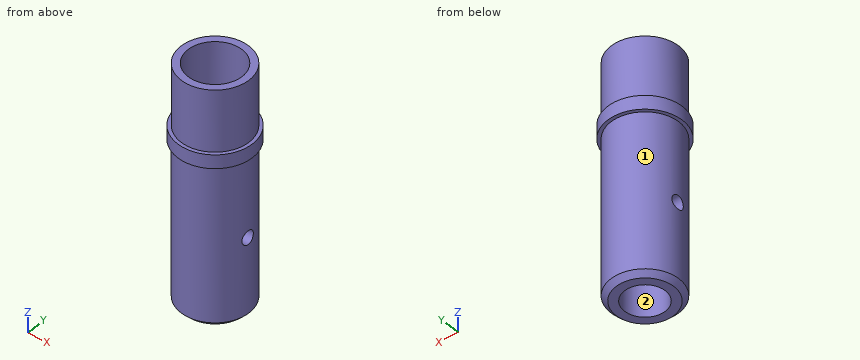
from build123d import *

# Parameters (mm, degrees)
SZKIC1_R                    = 10
SZKIC1_R_2                  = 7.9375
DODANIE_WYCI_GNI_CIE1_DEPTH = 18
SZKIC2_R                    = 11
SZKIC2_R_2                  = 7.9375
DODANIE_WYCI_GNI_CIE2_DEPTH = 4
SZKIC3_R                    = 10
SZKIC3_R_2                  = 6
DODANIE_WYCI_GNI_CIE3_DEPTH = 47
SFAZOWANIE1_SIZE            = 1.5
SZKIC6_R                    = 2
WYTNIJ_WYCI_GNI_CIE1_DEPTH  = 15


with BuildPart() as part:
    # Szkic1 → Dodanie-wyciągnięcie1 (new body)
    with BuildSketch(Plane.XY):
        Circle(SZKIC1_R)
        Circle(SZKIC1_R_2, mode=Mode.SUBTRACT)
    extrude(amount=DODANIE_WYCI_GNI_CIE1_DEPTH)

    # Szkic2 → Dodanie-wyciągnięcie2 (add)
    with BuildSketch(Plane(origin=(0, 0, 0), x_dir=(-1, 0, 0), z_dir=(0, 0, -1))):
        Circle(SZKIC2_R)
        Circle(SZKIC2_R_2, mode=Mode.SUBTRACT)
    extrude(amount=DODANIE_WYCI_GNI_CIE2_DEPTH)

    # Szkic3 → Dodanie-wyciągnięcie3 (add)
    with BuildSketch(Plane(origin=(0, 0, -4), x_dir=(-1, 0, 0), z_dir=(0, 0, -1))):
        Circle(SZKIC3_R)
        Circle(SZKIC3_R_2, mode=Mode.SUBTRACT)
    extrude(amount=DODANIE_WYCI_GNI_CIE3_DEPTH)

    # Sfazowanie1
    sfazowanie1_edges = [part.edges().sort_by_distance(p)[0] for p in [
        (10, 0, -51),
    ]]
    chamfer(sfazowanie1_edges, length=SFAZOWANIE1_SIZE)

    # Szkic6 → Wytnij-wyciągnięcie1 (cut, symmetric)
    with BuildSketch(Plane(origin=(0, 0, 0), x_dir=(0, 0, -1), z_dir=(1, 0, 0))):
        with Locations((27.5, 0)):
            Circle(SZKIC6_R)
    extrude(amount=WYTNIJ_WYCI_GNI_CIE1_DEPTH, both=True, mode=Mode.SUBTRACT)


solid = part.part
Verification items for the finished model (mm, model axes). Face numbers are marked on the shaded views. Coordinates: 2 decimals unless noted, no trailing zeros. Order: outer loops, then holes, each group sorted by start corner. A loop starts at its lowest first (then second) coordinate and runs counter-clockwise, first axis right, second up. Notation, with made-up numbers: (66.25, -38) -> (107.25, -38) arc R31 cw to (107.25, -12) -> close; hole circle Ø8 at (58.25, -39). An arc over 180 degrees is marked (long way). Put each result on its own line as item: value. Start each with the question number.
1. Cross-section at A-A, the plane y = 0. Count the separate pieces of the cut face and the enclosed holes in it, then the cut area to 4 significant figures.
2. Cross-section at C-C, the plane z = -27.5. Record the boundary of the cut face in (x, y), then the cut area to 3 significant figures.
3. Go/stop test with flat-tipped pins: pin 1 Ø2 at (x, z) = (-5, -10) entering from +Y; pin 2 Ø6 at (x, y) = (-2.5, 2) entering from +Z; pin 3 Ø4 at (x, z) = (-4, -4) entering from -Y. Record where each tip stops, or that it passes through.
4. Material ranges on L1, parallel to Y at x = 0, z = -28.5; L2, parallel to Y at x = 0, z = -1.25; L3, parallel to Z at x = -4.75, y = -9.5, recorded low to high. Write a range as [from, to].
5. Cross-section at B-B, the plane x = 0. Record the boundary of the cut face in (y, z), then the cut area to 4 significant figures.
6. Mould release check, pull along Y, two halves, no side actions. Record for the marked faces 1 and 2: released by +Y, released by -Y, zero draft, split by the parting line, or undercut.
7. Cross-section at D-D, the plane z = -45. Record the boundary of the cut face in (x, y), then the cut area to 3 significant figures.
Computed:
1. separate pieces: 4
1. enclosed holes: 0
1. area: 440.5 mm2
2. outline: (-9.8, -2) arc R10 ccw to (9.8, -2) -> (5.66, -2) arc R6 cw to (-5.66, -2) -> close; (-9.8, 2) -> (-5.66, 2) arc R6 cw to (5.66, 2) -> (9.8, 2) arc R10 ccw to start
2. area: 169 mm2
3. pin 1: y = 9.17
3. pin 2: z = -4
3. pin 3: y = -10.82
4. L1: [-10, -6], [6, 10]
4. L2: [-11, -7.94], [7.94, 11]
4. L3: [-4, 0]
5. outline: (-11, -4) -> (-10, -4) -> (-10, -49.5) -> (-8.5, -51) -> (-6, -51) -> (-6, -4) -> (-7.94, -4) -> (-7.94, 18) -> (-10, 18) -> (-10, 0) -> (-11, 0) -> close; (6, -51) -> (8.5, -51) -> (10, -49.5) -> (10, -4) -> (11, -4) -> (11, 0) -> (10, 0) -> (10, 18) -> (7.94, 18) -> (7.94, -4) -> (6, -4) -> close
5. area: 472.5 mm2
6. face 1: split by the parting line
6. face 2: undercut
7. outline: circle Ø20 at (0, 0); hole circle Ø12 at (0, 0)
7. area: 201 mm2
